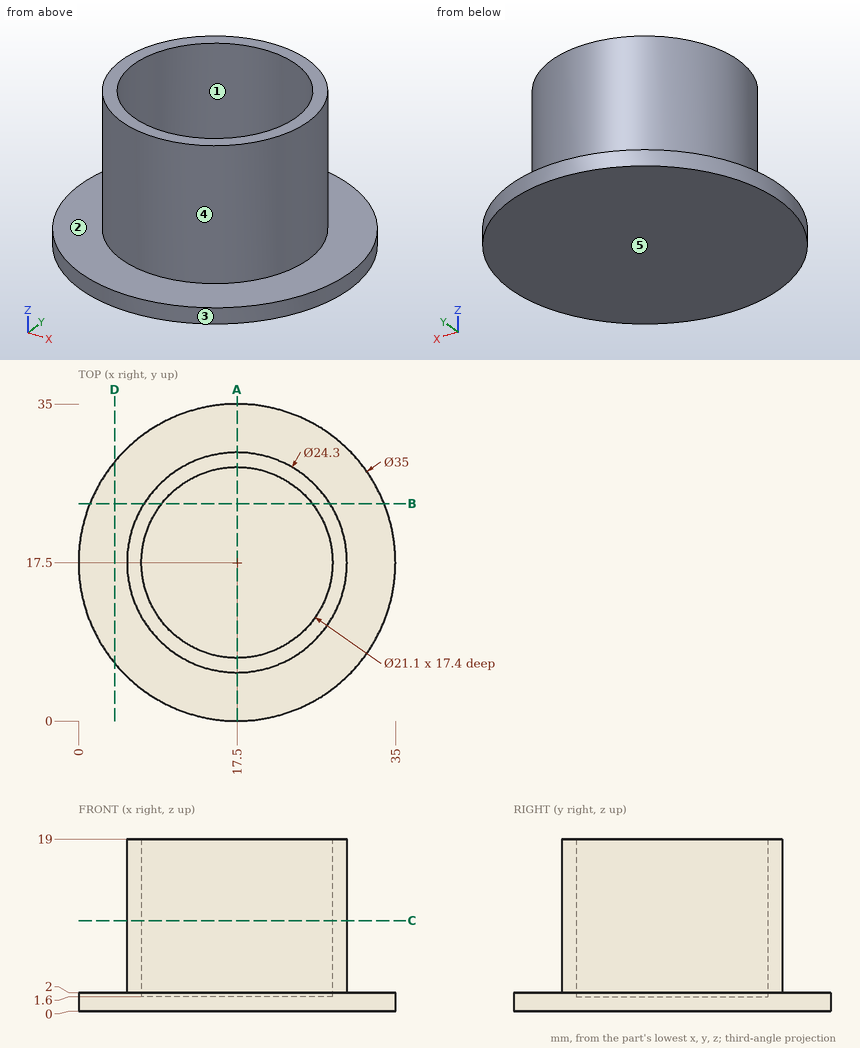
Geometry: see drawing. Coordinates: mm, zero at the bounding-box minimum. A direction names the side the tool comes from. Round coordinates to 2 decimals unless told otherwise and drop trailing zeros. Write each loop counter-clockwise with the first axis right and the second up, starting at its lowest first coordinate (ties: lowest second). Pieces come first, ordered by that corner, then holes. Notation, with made-up numbers: M 10,0.5 L 65,0.5 A21 ccw 65,18.5 Z; hole C 34.5,-37.75 d11. An arc over 180 degrees is marked long. Answer as a JSON object with one key per item and string values. Group by question number.
(1) Mould query, pull axis Y, two halves, no side actions, for the marked faces 1, 2 and 3. Classes: +Y half, -Y half, draft (parallel to the pull), parting line (faces both ways), or undercut.
(2) First-contact query: pin 1 (10 mm diameter, centred on y = 29, z = 3.5, fed in from -X); pin 2 (8 mm diameter, centred on x = 8.5, z = 4.5, fed in from -Y); pin 3 (4 mm diameter, centred on y = 18.5, z = 13, fed in from -X). Flat tips, straight axial feed; report the tip coordinate or a pass-through.
(3) Section query D-D on x = 4. Output: boundary loops of the cut face in (y, z).
(4) Ray query, line 1 (Y direction, x = 17.5, z = 9.5); line 2 (X direction, y = 21.5, z = 18.25); line 3 (X direction, y = 16.5, z = 9). Return the intervals inside material, ascending. Write a range as [from, to].
(5) Section query A-A on x = 17.5. Output: boundary loops of the cut face in (y, z).
(6) Section query C-C on z = 10. Output: boundary loops of the cut face in (x, y), then the cut area to 3 significant figures.
(7) Section query B-B on y = 24. Output: boundary loops of the cut face in (x, z).
(8) Reachability of the marked faces 4 and 5 from +Z, -Z, +X, -X, +Y, -Y: full face, straight path, thin tool, end or side. Return the list, or none.
Computed values:
{
 "1": {"face 1": "undercut", "face 2": "draft", "face 3": "parting line"},
 "2": {"pin 1": "x = 1.35", "pin 2": "y = 1.02", "pin 3": "x = 5.35"},
 "3": {"outline": "M 6.36,0 L 28.64,0 L 28.64,2 L 6.36,2 Z"},
 "4": {"line 1": "[5.35, 6.95], [28.05, 29.65]", "line 2": "[6.03, 7.74], [27.26, 28.97]", "line 3": "[5.39, 7], [28, 29.61]"},
 "5": {"outline": "M 0,0 L 35,0 L 35,2 L 29.65,2 L 29.65,19 L 28.05,19 L 28.05,1.6 L 6.95,1.6 L 6.95,19 L 5.35,19 L 5.35,2 L 0,2 Z"},
 "6": {"outline": "C 17.5,17.5 d24.3; hole C 17.5,17.5 d21.1", "area": "114 mm^2"},
 "7": {"outline": "M 1.25,0 L 33.75,0 L 33.75,2 L 27.77,2 L 27.77,19 L 25.81,19 L 25.81,1.6 L 9.19,1.6 L 9.19,19 L 7.23,19 L 7.23,2 L 1.25,2 Z"},
 "8": {"face 4": "+Z", "face 5": "-Z, +X, -X, +Y, -Y"}
}
